The model under review builds one solid part; all positions refer to its coordinate system, in mm. Face numbers are marked on the shaded views. A direction names the side the tool comes from. Round coordinates to 2 decimals unless told otherwise and drop trailing zeros. Loops run counter-clockwise (first coordinate to the right, second up) from the corner with the lowest first, then second, coordinate; pieces in that order, holes last. Notation, with made-up numbers: M 32,77 L 56,77 A26 cw 56,112 Z; hole C 70.5,-9 d8. An arc over 180 degrees is marked long. Answer as a JSON object with one key per item and string values. Group by question number.
Item 1: Insertion check: P1, Ø1.5, axis at y = 4.5, z = 14, coming from the -X side; P2, Ø3, axis at y = -13.5, z = 12, coming from the -X side; P3, Ø10, axis at x = 44, z = 9, coming from the -Y side. Each pin has a flat end and moves straight along its axis. Give the tip position at first contact, or say it passes through.
Item 2: Consider section A-A (z = -7.5). Give the boundary of the cut face in (x, y) (3 decimals), and give its area (3 significant figures).
Item 3: Tool access review of the marked faces 4 and 5: name each direction out of +Z, -Z, +X, -X, +Y, -Y from which nothing blocks a thin tool from reaching the whole face with its end or side.
Item 4: Consider section C-C (x = -2). Give the boundary of the cut face in (y, z) (1 decimal), and give its area (3 significant figures).
Item 5: To check wall thickness, follow line 1 (Z direction, x = 0, y = 11.5); line 2 (Z direction, x = 0, y = 44.5); line 3 (Y direction, x = 46.5, z = 0.5). State the ranges of each line that lie inside material, in increasing order.
Item 6: Consider section D-D (y = 37). Give the boundary of the cut face in (x, z).
Item 7: The part is to be moulded in two halves that separate along X. For the marked faces 1, 2 and 3, say which applies: +X half, -X half, draft (parallel to the pull), parting line (faces both ways), or undercut.
Autodesk Inventor part; units mm, degrees
ref_plane "Work Plane1" through (53.848, 0, 0) normal (1, 0, 0) x (0, 1, 0)
ref_plane "XZ Plane" through (0, 0, 0) normal (0, 1, 0) x (-1, 0, 0)
ref_plane "XY Plane" through (0, 0, 0) normal (0, 0, 1) x (1, 0, 0)
sketch "Sketch1" plane through (0, 0, 0) normal (0, 1, 0) x (-1, 0, 0)
  circle A0 centre (0, 0) radius 21.209
  circle A1 centre (0, 0) radius 24.892
  dimension "d0" = 42.418
  dimension "d1" = 49.784
extrude "Extrusion1" add sketch "Sketch1" along normal mid plane 107.696
sketch "Sketch4" plane through (0, 0, 0) normal (0, 1, 0) x (-1, 0, 0)
  circle A0 centre (0, 0) radius 17.526
  circle A1 centre (0, 0) radius 21.209
  circle A2 centre (0, 0) radius 24.892
  dimension "d9" = 35.052
extrude "Extrusion4" add sketch "Sketch4" along normal mid plane 44.45 contours A1
ref_plane "Work Plane1" through (53.848, 0, 0) normal (1, 0, 0) x (0, 1, 0)
sketch "Sketch2" plane through (53.848, 0, 0) normal (1, 0, 0) x (0, 1, 0)
  line L0 (-53.848, 24.892) -> (-53.848, -24.892)
  line L1 (53.848, -24.892) -> (53.848, 24.892)
  circle A0 centre (0, 0) radius 24.892
  line L2 (-53.848, 24.892) -> (53.848, 24.892)
extrude "Extrusion2" add sketch "Sketch2" against normal up to next
sketch "Sketch3" plane through (53.848, 0, 0) normal (1, 0, 0) x (0, 0, -1)
  line L0 (-21.209, -53.848) -> (-21.209, -22.225)
  circle A0 centre (0, 0) radius 21.209
extrude "Extrusion3" cut sketch "Sketch3" against normal blind 31.623
sketch "Sketch5" plane through (22.225, 0, 0) normal (1, 0, 0) x (0, 0, -1)
  line L0 (-17.526, -22.225) -> (-17.526, 22.225)
  circle A0 centre (0, 0) radius 17.526
extrude "Extrusion5" cut sketch "Sketch5" against normal up to next
properties part number "Piping_Tee_1.25in" material "PVC-Piping"
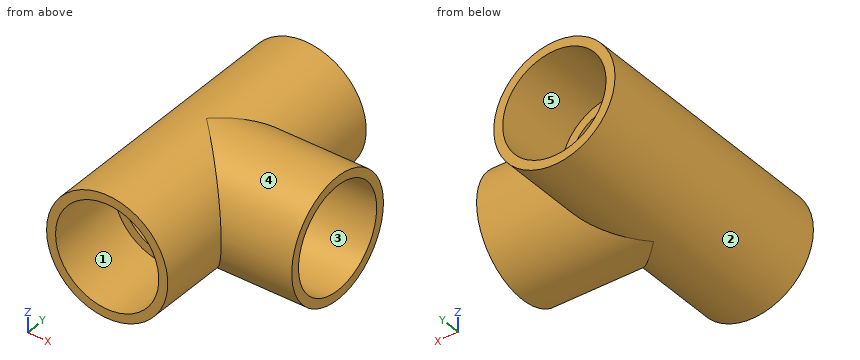
Geometry results:
{
 "1": {"P1": "stops at x = -21.07", "P2": "stops at x = -22.57", "P3": "stops at y = -24.57"},
 "2": {"outline": "M -23.735,-53.848 L -19.839,-53.848 L -19.839,-22.225 L -15.84,-22.225 L -15.84,22.225 L -19.839,22.225 L -19.839,53.848 L -23.735,53.848 Z; M 15.84,-22.225 L 19.839,-22.225 L 19.839,-53.848 L 23.735,-53.848 L 23.735,-23.735 L 53.848,-23.735 L 53.848,-19.839 L 22.225,-19.839 L 22.225,-15.84 L 15.84,-15.84 Z; M 15.84,15.84 L 22.225,15.84 L 22.225,19.839 L 53.848,19.839 L 53.848,23.735 L 23.735,23.735 L 23.735,53.848 L 19.839,53.848 L 19.839,22.225 L 15.84,22.225 Z", "area": "1,170 mm^2"},
 "3": {"face 4": "+X", "face 5": "+Y"},
 "4": {"outline": "M -53.8,-24.8 L 53.8,-24.8 L 53.8,-21.1 L 22.2,-21.1 L 22.2,-17.4 L -22.2,-17.4 L -22.2,-21.1 L -53.8,-21.1 Z; M -53.8,21.1 L -22.2,21.1 L -22.2,17.4 L 22.2,17.4 L 22.2,21.1 L 53.8,21.1 L 53.8,24.8 L -53.8,24.8 Z", "area": "1,130 mm^2"},
 "5": {"line 1": "z = -24.89 to -17.53, 17.53 to 24.89", "line 2": "z = -24.89 to -21.21, 21.21 to 24.89", "line 3": "y = -24.89 to -21.2, 21.2 to 24.89"},
 "6": {"outline": "C 0,0 d49.78; hole C 0,0 d42.42"},
 "7": {"face 1": "undercut", "face 2": "parting line", "face 3": "draft"}
}
